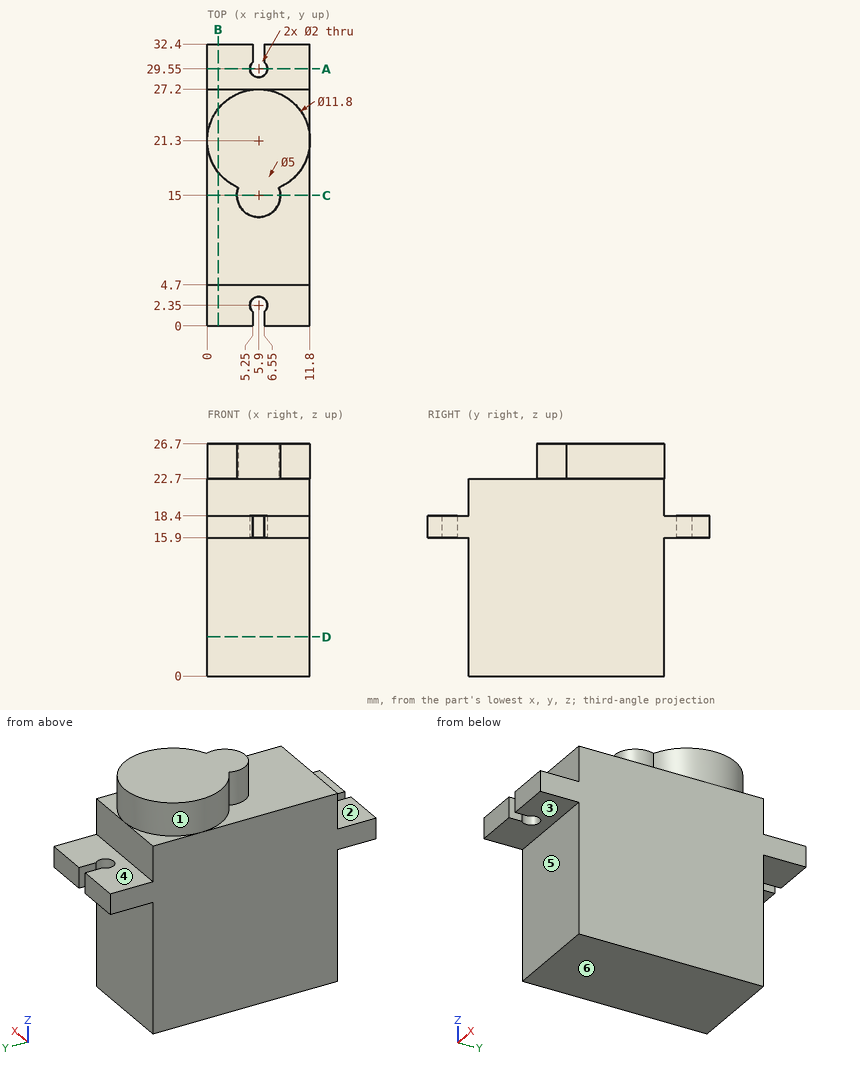
Verification items for this drawing (mm, ordinates from the low corner). A direction names the side the tool comes from. Round coordinates to 2 decimals unless told otherwise and drop trailing zeros. Loops run counter-clockwise (first coordinate to the right, second up) from the corner with the lowest first, then second, coordinate; pieces in that order, holes last. Notation, with made-up numbers: (32, -12) - (50, -12) arc R20 ccw to (50, -4) - close; hole circle Ø4 at (62.5, 86.25). An arc over 180 degrees is marked (long way). Answer as CSV lines item,"result". Start each with the question number.
Item 1: Scan lines: line 1 (X direction, y = 2.35, z = 17.1); line 2 (Y direction, x = 1, z = 13); line 3 (Y direction, x = 5.9, z = 17.5). Record each from-to range of solid material in increasing order. Write a range as [from, to].
Item 2: Section check C-C (y = 15). Record the boundary of the cut face in (x, z), and give its area (3 significant figures).
Item 3: Section check D-D (z = 4.5). Record the boundary of the cut face in (x, y).
Item 4: Set-up check for the marked faces 1, 2 and 3: record each of +Z, -Z, +X, -X, +Y, -Y from which the full face is reachable in a straight line by a thin tool's end or side.
Item 5: Depth check by flat-ended pin: P1, Ø1.4, axis at x = 7.5, y = 2.5, coming from the +Z side; P2, Ø1.6, axis at x = 4, y = 28.5, coming from the -Z side; P3, Ø5, axis at x = 8.5, z = 21.5, coming from the +Y side. Enter the tip coordinate at first touch or a pass-through.
Item 6: Section check B-B (x = 1.25). Record the boundary of the cut face in (y, z), and give its area (3 significant figures).
Item 7: Release check for a two-part mould opening along Z. For the marked faces 4, 5 and 6 record: +Z half, -Z half, draft (parallel to the pull), parting line (faces both ways), or undercut.
Item 8: Section check A-A (y = 29.55). Record the boundary of the cut face in (x, z).
Report:
1,line 1,"x = [0, 4.9], [6.9, 11.8]"
1,line 2,"y = [4.7, 27.2]"
1,line 3,"y = [3.35, 28.55]"
2,outline,"(0, 0) - (11.8, 0) - (11.8, 22.7) - (8.4, 22.7) - (8.4, 26.7) - (3.4, 26.7) - (3.4, 22.7) - (0, 22.7) - close"
2,area,"288 mm2"
3,outline,"(0, 4.7) - (11.8, 4.7) - (11.8, 27.2) - (0, 27.2) - close"
4,face 1,"+Z"
4,face 2,"+Z, +X, -X, -Y"
4,face 3,"-Z, +X, -X, -Y"
5,P1,"stops at z = 18.4"
5,P2,"stops at z = 15.9"
5,P3,"stops at y = 27.2"
6,outline,"(0, 15.9) - (4.7, 15.9) - (4.7, 0) - (27.2, 0) - (27.2, 15.9) - (32.4, 15.9) - (32.4, 18.4) - (27.2, 18.4) - (27.2, 22.7) - (24.93, 22.7) - (24.93, 26.7) - (17.67, 26.7) - (17.67, 22.7) - (4.7, 22.7) - (4.7, 18.4) - (0, 18.4) - close"
6,area,"565 mm2"
7,face 4,"+Z half"
7,face 5,"draft"
7,face 6,"-Z half"
8,outline,"(0, 15.9) - (4.9, 15.9) - (4.9, 18.4) - (0, 18.4) - close; (6.9, 15.9) - (11.8, 15.9) - (11.8, 18.4) - (6.9, 18.4) - close"
